Autodesk Inventor part; units mm, degrees
ref_plane "YZ Plane" through (0, 0, 0) normal (1, 0, 0) x (0, 1, 0)
ref_plane "XZ Plane" through (0, 0, 0) normal (0, 1, 0) x (-1, 0, 0)
ref_plane "XY Plane" through (0, 0, 0) normal (0, 0, 1) x (1, 0, 0)
sketch "Sketch1" plane through (0, 0, 0) normal (0, 0, 1) x (1, 0, 0)
  line L0 (0, 0) -> (-14, 0) construction
  circle A0 centre (-14, 0) radius 4
  circle A1 centre (0, 0) radius 4
  line L1 (12, -9) -> (-26, -9)
  line L2 (-26, -9) -> (-26, 9)
  line L3 (-26, 9) -> (12, 9)
  line L4 (12, 9) -> (12, -9)
  line L5 (12, -9) -> (-26, 9) construction
  line L6 (-26, -9) -> (12, 9) construction
  point P0 (-7, 0)
  dimension "d0" = 8
  dimension "d1" = 14
  dimension "d2" = 12
  dimension "d3" = 18
  dimension "d13" = 38
extrude "Extrusion1" add sketch "Sketch1" along normal blind 10
sketch "Sketch2" plane through (-26, 9, 0) normal (0, 1, 0) x (1, 0, 0)
  circle A0 centre (19, -5) radius 2.5
  line L0 (19, -5) -> (0, -5) construction
  line L1 (0, 0) -> (0, -10) construction
  point P0 (26, 0)
  dimension "d6" = 5
  dimension "d17" = 19
extrude "Extrusion2" cut sketch "Sketch2" against normal through all
fillet "Fillet1" radius 6 4 edges at (12, 9, 5) (-26, 9, 5) (-26, -9, 5) (12, -9, 5)
sketch "Sketch3" plane through (0, 0, 10) normal (0, 0, 1) x (1, 0, 0)
  line L0 (-20, -9) -> (6, -9)
  circle A0 centre (0, 0) radius 4
  circle A1 centre (-14, 0) radius 4
  line L1 (-14, 0) -> (0, 0) construction
  line L2 (0, -0.75) -> (-14, -0.75)
  line L3 (-14, -0.75) -> (-14, 0.75)
  line L4 (-14, 0.75) -> (0, 0.75)
  line L5 (0, 0.75) -> (0, -0.75)
  line L6 (0, -0.75) -> (-14, 0.75) construction
  line L7 (-14, -0.75) -> (0, 0.75) construction
  point P0 (-7, 0)
  dimension "d10" = 1.5
extrude "Extrusion3" cut sketch "Sketch3" against normal through all contours L4 L5 L2 A0 | A0 L2 A1 L4 | A1 L2 L3 L4 picked at (-1.3307, -0.0838) picked at (-12.6667, 0)
sketch "Sketch4" plane through (0, 0, 10) normal (0, 0, 1) x (1, 0, 0)
  line L0 (-10.0709, 0.75) -> (-3.9291, 0.75) construction
  arc A0 (-3.9291, -0.75) -> (-3.9291, 0.75) centre (0, 0) ccw construction
  line L1 (-3.9291, -0.75) -> (-10.0709, -0.75) construction
  arc A1 (-10.0709, 0.75) -> (-10.0709, -0.75) centre (-14, 0) ccw construction
  arc A2 (6, -9) -> (12, -3) centre (6, -3) ccw construction
  line L2 (12, -3) -> (12, 3) construction
  arc A3 (12, 3) -> (6, 9) centre (6, 3) ccw construction
  line L3 (6, 9) -> (-20, 9) construction
  arc A4 (-20, 9) -> (-26, 3) centre (-20, 3) ccw construction
  line L4 (-26, 3) -> (-26, -3) construction
  arc A5 (-26, -3) -> (-20, -9) centre (-20, -3) ccw construction
  line L5 (-20, -9) -> (6, -9) construction
  line L6 (-9.2375, -4.7625) -> (-18.7625, -4.7625)
  line L7 (-18.7625, -4.7625) -> (-18.7625, 4.7625)
  line L8 (-18.7625, 4.7625) -> (-9.2375, 4.7625)
  line L9 (-9.2375, 4.7625) -> (-9.2375, -4.7625)
  line L10 (-9.2375, -4.7625) -> (-18.7625, 4.7625) construction
  line L11 (-18.7625, -4.7625) -> (-9.2375, 4.7625) construction
  dimension "d14" = 9.525
extrude "Extrusion4" [suppressed]
properties part number "crank web2"
Check sheet for the modelled part. Datum: model origin and axes. Units: mm. A direction names the side the tool comes from. Give positions to 0.01 mm unless a question says otherwise; leave off trailing zeros. Write each loop counter-clockwise with the first axis right and the second up, starting at its lowest first coordinate (ties: lowest second). Pieces come first, ordered by that corner, then holes. Notation, with made-up numbers: (72.5, 35.5) - (91.5, 35.5) arc R9 ccw to (91.5, 48.5) - close; hole circle Ø11 at (-4, 62). An arc over 180 degrees is marked (long way). Answer as a JSON object with one key per item and string values. Group by question number.
1) Release check for a two-part mould opening along Y. For faces 1 (the face through (-4, -9, 5)), 2 (the face through (-8.4, 0.75, 7.3)), 3 (the face through (12, 0, 5)) record: pulls with the +Y half, pulls with the -Y half, needs draft (parallel to the pull), parting line crosses it, or undercut.
2) Sectioned sample at B-B (z = 7). Record the cut outline in (x, y), then the cut area to 3 significant figures.
3) Thickness scan on probe 1 along Y at (x, z) = (0, 3); probe 2 along X at (y, z) = (0, 7); probe 3 along Z at (x, y) = (-7, 6.75). Record the ranges inside material, lowest first. Write a range as from..to.
4) Depth check by flat-ended pin: P1, Ø4.5, axis at x = -7, z = 5, coming from the -Y side. Enter the tip coordinate at first touch or a pass-through.
5) Sectioned sample at A-A (y = 0). Record the cut outline in (x, z).
6) Access from +Z, -Z, +X, -X, +Y, -Y to the whole of each face (thin tool, end or side, straight path). Record for faces 4 (the face through (10.289, 7.196, 5.07)), 5 (the face through (-5.6, -0.75, 7.3)).
7) Sectioned sample at C-C (x = -7). Record the cut outline in (y, z).
8) Sectioned sample at D-D (x = 0). Record the cut outline in (y, z), then the cut area to 3 significant figures.
Geometry results:
{
 "1": {"face 1": "pulls with the -Y half", "face 2": "undercut", "face 3": "needs draft"},
 "2": {"outline": "(-26, -3) arc R6 ccw to (-20, -9) - (-8.5, -9) - (-8.5, -0.75) - (-10.07, -0.75) arc R4 cw (long way) to (-10.07, 0.75) - (-8.5, 0.75) - (-8.5, 9) - (-20, 9) arc R6 ccw to (-26, 3) - close; (-5.5, -9) - (6, -9) arc R6 ccw to (12, -3) - (12, 3) arc R6 ccw to (6, 9) - (-5.5, 9) - (-5.5, 0.75) - (-3.93, 0.75) arc R4 cw (long way) to (-3.93, -0.75) - (-5.5, -0.75) - close", "area": "494 mm^2"},
 "3": {"probe 1": "y = -9..-4, 4..9", "probe 2": "x = -26..-18, 4..12", "probe 3": "z = 0..2.5, 7.5..10"},
 "4": {"P1": "passes through"},
 "5": {"outline": "(-26, 0) - (-18, 0) - (-18, 10) - (-26, 10) - close; (4, 0) - (12, 0) - (12, 10) - (4, 10) - close"},
 "6": {"face 4": "+Z, -Z, +X, +Y", "face 5": "+Z, -Z"},
 "7": {"outline": "(-9, 0) - (-0.75, 0) - (-0.75, 2.5) - (-9, 2.5) - close; (-9, 7.5) - (-0.75, 7.5) - (-0.75, 10) - (-9, 10) - close; (0.75, 0) - (9, 0) - (9, 2.5) - (0.75, 2.5) - close; (0.75, 7.5) - (9, 7.5) - (9, 10) - (0.75, 10) - close"},
 "8": {"outline": "(-9, 0) - (-4, 0) - (-4, 10) - (-9, 10) - close; (4, 0) - (9, 0) - (9, 10) - (4, 10) - close", "area": "100 mm^2"}
}
